Source: CAD feature listing. Evaluate the final solid. Frame: model axes, mm. Coordinates: 2 decimals unless noted, no trailing zeros. Loops run counter-clockwise (first coordinate to the right, second up) from the corner with the lowest first, then second, coordinate; pieces in that order, holes last.
Item 1: Section query B-B, the plane z = 450. Return the cut outline in (x, y).
Item 2: Section query A-A, the plane y = 0. Return the cut outline in (x, z).
Item 3: Section query C-C, the plane z = 148.5. Return the cut outline in (x, y), then the cut area to 3 significant figures.
Item 4: Pin query (flat end, axial travel): pin 1 Ø3 at (y, z) = (15, 355) entering from +X. Return the tip coordinate at first contact, or that it passes through.
Item 5: Line query: probe 1 along Y at (x, z) = (24.05, 530); probe 2 along X at (y, z) = (4, 278). Output: solid intervals per line, ascending.
```python
from build123d import *

# Parameters (mm, degrees)
SKETCH1_W           = 50
SKETCH1_H           = 50
SKETCH1_W_2         = 47
SKETCH1_H_2         = 47
BOSS_EXTRUDE1_DEPTH = 900
SKETCH2_R           = 15
CUT_EXTRUDE1_DEPTH  = 59
CUT_EXTRUDE2_DEPTH  = 10
CUT_EXTRUDE3_DEPTH  = 10
SKETCH5_R           = 3
CUT_EXTRUDE4_DEPTH  = 55
SKETCH6_R           = 3.125
SKETCH6_R_2         = 5
CUT_EXTRUDE5_DEPTH  = 70
SKETCH7_R           = 2.5
CUT_EXTRUDE6_DEPTH  = 902.734439844


with BuildPart() as part:
    # Sketch1 → Boss-Extrude1 (new body)
    with BuildSketch(Plane.XY):
        Rectangle(SKETCH1_W, SKETCH1_H)
        Rectangle(SKETCH1_W_2, SKETCH1_H_2, mode=Mode.SUBTRACT)
    extrude(amount=BOSS_EXTRUDE1_DEPTH)

    # Sketch2 → Cut-Extrude1 (cut)
    with BuildSketch(Plane(origin=(25, 0, 0), x_dir=(0, 0, -1), z_dir=(1, 0, 0))):
        with Locations(Location((-450, 0, 0), (0, 0, 90))):
            Circle(SKETCH2_R)
    extrude(amount=-CUT_EXTRUDE1_DEPTH, mode=Mode.SUBTRACT)

    # Sketch3 → Cut-Extrude2 (cut)
    with BuildSketch(Plane(origin=(0, 25, 0), x_dir=(1, 0, 0), z_dir=(0, 1, 0))):
        with BuildLine():
            Line((14, -843), (14, -913.98611775))
            ThreePointArc((14, -913.98611775), (0, -927.98611775), (-14, -913.98611775))
            Line((-14, -913.98611775), (-14, -843))
            ThreePointArc((-14, -843), (0, -829), (14, -843))
        make_face()
    cut_extrude2 = extrude(amount=-CUT_EXTRUDE2_DEPTH, mode=Mode.SUBTRACT)

    # Sketch4 → Cut-Extrude3 (cut)
    with BuildSketch(Plane.XZ.offset(25)):
        with BuildLine():
            Line((-17.498938419, 850), (-17.498938419, 939.078503923))
            ThreePointArc((-17.498938419, 939.078503923), (0.001061581, 956.578503923), (17.501061581, 939.078503923))
            Line((17.501061581, 939.078503923), (17.501061581, 850))
            ThreePointArc((17.501061581, 850), (0.001061581, 832.5), (-17.498938419, 850))
        make_face()
    cut_extrude3 = extrude(amount=-CUT_EXTRUDE3_DEPTH, mode=Mode.SUBTRACT)

    # Sketch5 → Cut-Extrude4 (cut)
    with BuildSketch(Plane(origin=(25, 0, 0), x_dir=(0, 0, -1), z_dir=(1, 0, 0))):
        with Locations(Location((-882.5, 11, 0), (0, 0, 90))):
            Circle(SKETCH5_R)
        with Locations(Location((-882.5, -11, 0), (0, 0, 90))):
            Circle(SKETCH5_R)
        with Locations(Location((-816.5, -11, 0), (0, 0, 90))):
            Circle(SKETCH5_R)
        with Locations(Location((-816.5, 11, 0), (0, 0, 90))):
            Circle(SKETCH5_R)
    cut_extrude4 = extrude(amount=-CUT_EXTRUDE4_DEPTH, mode=Mode.SUBTRACT)

    # Mirror1: Cut-Extrude2, Cut-Extrude3, Cut-Extrude4 across plane
    add(cut_extrude2.mirror(Plane.XY.offset(450)), mode=Mode.SUBTRACT)
    add(cut_extrude3.mirror(Plane.XY.offset(450)), mode=Mode.SUBTRACT)
    add(cut_extrude4.mirror(Plane.XY.offset(450)), mode=Mode.SUBTRACT)

    # Sketch6 → Cut-Extrude5 (cut)
    with BuildSketch(Plane(origin=(0, 25, 0), x_dir=(1, 0, 0), z_dir=(0, 1, 0))):
        with Locations(Location((0, -694.2275, 0), (0, 0, 270))):
            Circle(SKETCH6_R)
        with Locations(Location((0, -739.8525, 0), (0, 0, 270))):
            Circle(SKETCH6_R)
        with Locations(Location((0, -717.04, 0), (0, 0, 270))):
            Circle(SKETCH6_R_2)
    cut_extrude5 = extrude(amount=-CUT_EXTRUDE5_DEPTH, mode=Mode.SUBTRACT)

    # Mirror2: Cut-Extrude5 across plane
    add(cut_extrude5.mirror(Plane.XY.offset(450)), mode=Mode.SUBTRACT)

    # Sketch7 → Cut-Extrude6 (cut, through all)
    with BuildSketch(Plane.ZY.offset(25)):
        with Locations(Location((355, 15, 0), (0, 0, 270))):
            Circle(SKETCH7_R)
        with Locations(Location((370, 15, 0), (0, 0, 90))):
            Circle(SKETCH7_R)
        with Locations(Location((370, -15, 0), (0, 0, 270))):
            Circle(SKETCH7_R)
        with Locations(Location((355, -15, 0), (0, 0, 90))):
            Circle(SKETCH7_R)
        with Locations(Location((545, -15, 0), (0, 0, 270))):
            Circle(SKETCH7_R)
        with Locations(Location((530, -15, 0), (0, 0, 90))):
            Circle(SKETCH7_R)
        with Locations(Location((530, 15, 0), (0, 0, 270))):
            Circle(SKETCH7_R)
        with Locations(Location((545, 15, 0), (0, 0, 90))):
            Circle(SKETCH7_R)
    extrude(amount=-CUT_EXTRUDE6_DEPTH, mode=Mode.SUBTRACT)


solid = part.part
```
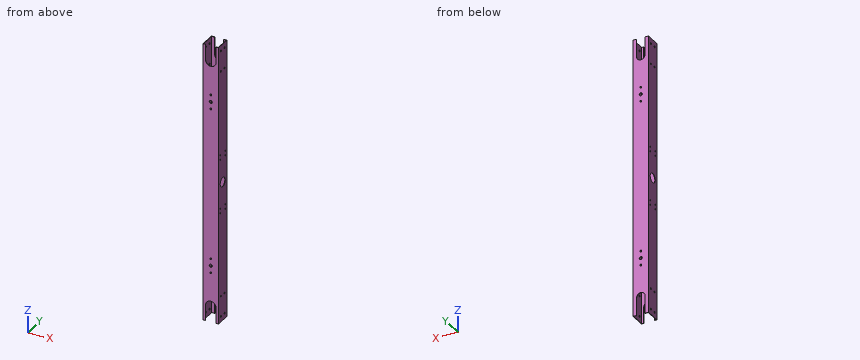
Verdict:
1. outline: (-25, -25) - (25, -25) - (25, -15) - (23.5, -15) - (23.5, -23.5) - (-23.5, -23.5) - (-23.5, -15) - (-25, -15) - close; (-25, 15) - (-23.5, 15) - (-23.5, 23.5) - (23.5, 23.5) - (23.5, 15) - (25, 15) - (25, 25) - (-25, 25) - close
2. outline: (-25, 0) - (-23.5, 0) - (-23.5, 435) - (-25, 435) - close; (-25, 465) - (-23.5, 465) - (-23.5, 900) - (-25, 900) - close; (23.5, 0) - (25, 0) - (25, 435) - (23.5, 435) - close; (23.5, 465) - (25, 465) - (25, 900) - (23.5, 900) - close
3. outline: (-25, -25) - (25, -25) - (25, 25) - (-25, 25) - close; hole (-23.5, -23.5) - (23.5, -23.5) - (23.5, 23.5) - (-23.5, 23.5) - close
3. area: 291 mm2
4. pin 1: passes through
5. probe 1: y = -25 to -17.5, -12.5 to 12.5, 17.5 to 25
5. probe 2: x = -25 to -23.5, 23.5 to 25
